from build123d import *

# Parameters (mm, degrees)
F0_R      = 22.5
F1_DEPTH  = 25
F2_R      = 22.5
F2_R_2    = 20
F3_DEPTH  = 5
F1_FACE_R = 20
F7_DEPTH  = 10
F6_R      = 12.5
F8_DEPTH  = 30
F10_DEPTH = 25


with BuildPart() as f1:
    # F0 (on Top) → F1 (new body)
    with BuildSketch(Plane.XY):
        Circle(F0_R)
    extrude(amount=F1_DEPTH)

    # F2 (on face) → F3 (cut)
    with BuildSketch(Plane(origin=(0, 0, 0), x_dir=(1, 0, 0), z_dir=(0, 0, -1))):
        Circle(F2_R)
        Circle(F2_R_2, mode=Mode.SUBTRACT)
    extrude(amount=-F3_DEPTH, mode=Mode.SUBTRACT)

    # F4 (on Front) → F5 (revolve, cut)
    with BuildSketch(Plane.XZ):
        Polygon((-22.5, 30), (-22.5, 10), (-17.5, 30), align=None)
    revolve(axis=Axis((0, 0, 15), (0, 0, 1)), mode=Mode.SUBTRACT)

    # F1_face (on face) → F7 (join)
    with BuildSketch(Plane(origin=(0, 0, 0), x_dir=(1, 0, 0), z_dir=(0, 0, -1))):
        Circle(F1_FACE_R)
    extrude(amount=F7_DEPTH)

    # F6 (on face) → F8 (cut)
    with BuildSketch(Plane.XY.offset(25)):
        Circle(F6_R)
    extrude(amount=-F8_DEPTH, mode=Mode.SUBTRACT)

    # F9 (on Front) → F10 (cut, symmetric)
    with BuildSketch(Plane.XZ):
        Polygon((2.5, -2.5), (0, -2.5), (0, -5), (0, -7.5), (2.5, -7.5), align=None)
        Polygon((0, -5), (0, -2.5), (-2.5, -2.5), (-2.5, -7.5), (0, -7.5), align=None)
    extrude(amount=F10_DEPTH, both=True, mode=Mode.SUBTRACT)


solid = f1.part
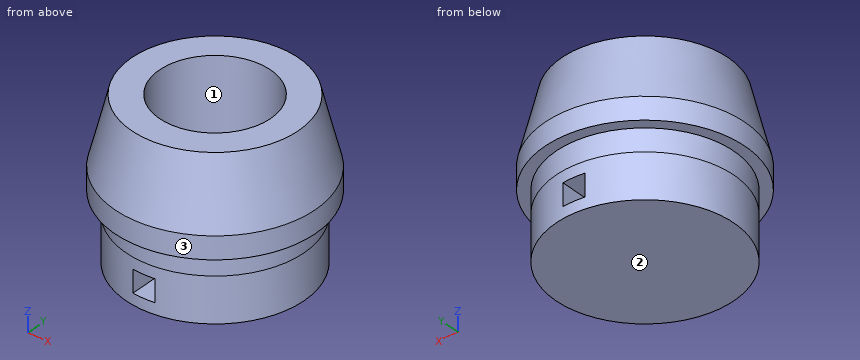
Source: CAD feature listing. Evaluate the final solid. Frame: model axes, mm. Face numbers are marked on the shaded views. Round coordinates to 2 decimals unless told otherwise and drop trailing zeros. Loops run counter-clockwise (first coordinate to the right, second up) from the corner with the lowest first, then second, coordinate; pieces in that order, holes last. Notation, with made-up numbers: M 69,46.5 L 91,46.5 A21 ccw 91,62.5 Z; hole C 80,-17 d2. An arc over 180 degrees is marked long. Answer as CSV lines item,"result".
Q1. Cut plane B-B (y = 0). Return the cut outline in (x, z).
Verdict:
outline,"M -22.5,5 L -20,5 L -20,-10 L 20,-10 L 20,5 L 22.5,5 L 22.5,10 L 18.75,25 L 12.5,25 L 12.5,-5 L 2.5,-5 L 2.5,-7.5 L -2.5,-7.5 L -2.5,-5 L -12.5,-5 L -12.5,25 L -18.75,25 L -22.5,10 Z"
Q2. Cut plane D-D (z = 7.5). Return the cut outline in (x, y).
Verdict:
outline,"C 0,0 d45; hole C 0,0 d25"
Q3. Line query: line 1 along Y through (x, z) = (0, 1); line 2 along X through (y, z) = (0, 6). Output: solid intervals per line, ascending.
Verdict:
line 1,"y = -20 to -12.5, 12.5 to 20"
line 2,"x = -22.5 to -12.5, 12.5 to 22.5"
Q4. Pull-direction query (X, two-part tool) for the marked faces 1, 2 and 3; classes: +X half, -X half, draft (parallel to the pull), parting line (faces both ways), or undercut.
Verdict:
face 1,"undercut"
face 2,"draft"
face 3,"parting line"
Q5. Contact query for flat-ended pins moving along their axis: pin 1 (2 mm diameter, centred on x = 1.5, z = 10, fed in from -Y); pin 2 (5.5 mm diameter, centred on y = 9, z = -5.5, fed in from -X); pin 3 (6 mm diameter, centred on x = -9.5, z = -2.5, fed in from +Y). Output: stop coordinate, or through.
Verdict:
pin 1,"stops at y = -22.49"
pin 2,"stops at x = -19"
pin 3,"stops at y = 18.91"
Q6. Cut plane C-C (z = 2). Return the cut outline in (x, y), plus the area to 3 significant figures.
Verdict:
outline,"C 0,0 d40; hole C 0,0 d25"
area,"766 mm^2"
Q7. Cut plane A-A (x = 0). Return the cut outline in (y, z), plus the area to 3 significant figures.
Verdict:
outline,"M -22.5,5 L -20,5 L -20,-2.5 L -12.5,-2.5 L -12.5,25 L -18.75,25 L -22.5,10 Z; M -20,-10 L 20,-10 L 20,-7.5 L -20,-7.5 Z; M 12.5,-2.5 L 20,-2.5 L 20,5 L 22.5,5 L 22.5,10 L 18.75,25 L 12.5,25 Z"
area,"556 mm^2"
